The drawing under review shows one solid part. Ordinate dimensions are in mm from its lowest x, y, z. A direction names the side the tool comes from. Round coordinates to 2 decimals unless told otherwise and drop trailing zeros. Order: outer loops, then holes, each group sorted by start corner. A loop starts at its lowest first (then second) coordinate and runs counter-clockwise, first axis right, second up. Notation, with made-up numbers: (7.25, -24.5) -> (54.25, -24.5) arc R26 cw to (54.25, -6.5) -> close; hole circle Ø10 at (71, 0.25). An arc over 180 degrees is marked (long way). Put each result on its own line as item: value. Start each with the question number.
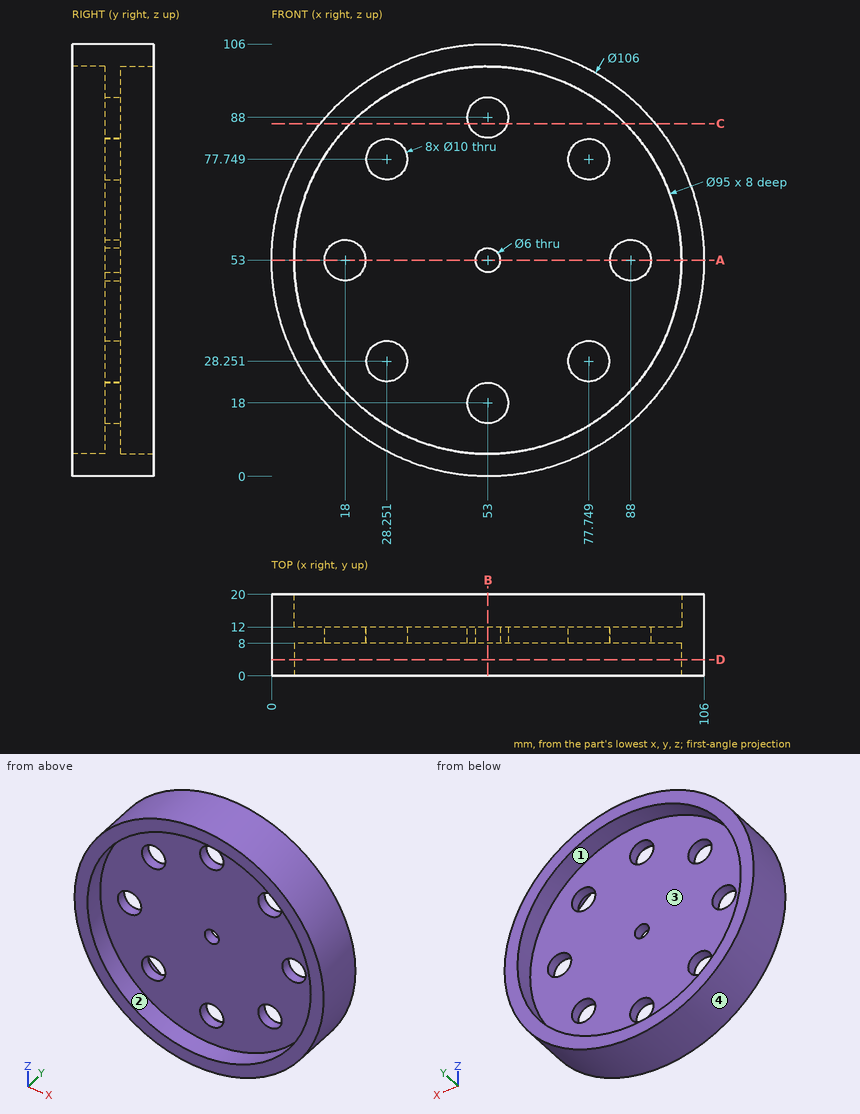
Item 1: Tool access review of the marked faces 1 and 2: name each direction out of +Z, -Z, +X, -X, +Y, -Y from which nothing blocks a thin tool from reaching the whole face with its end or side.
Item 2: Consider section B-B, the plane x = 53. Write out the cut boundary in (y, z).
Item 3: Consider section D-D, the plane y = 4. Write out the cut boundary in (x, z), plus the area to 3 significant figures.
Item 4: Mouldability with a two-part tool opening along X and no side actions: class the marked faces 3 and 4 as +X half, -X half, draft (parallel to the pull), parting line (faces both ways), or undercut.
Item 5: Consider section C-C, the plane z = 86.5. Write out the cut boundary in (x, y) (1 decimal).
Item 6: Consider section A-A, the plane z = 53. Write out the cut boundary in (x, y), plus the area to 3 significant figures.
Item 7: For L1, parallel to Z at x = 53, y = 9.15; L2, parallel to Z at x = 54, y = 17.5, list the stretches that pass through material, from the lowest coordinate up.
Item 8: Insertion check: pin 1 Ø6 at (y, z) = (13.5, 93) entering from -X; pin 2 Ø5 at (y, z) = (14, 24.5) entering from -X (1 decimal); pin 3 Ø7 at (x, z) = (53, 53) entering from +Y. Each pin has a flat end and moves straight along its axis. Give the tip position at first contact, or say it passes through.
Evaluation:
1. face 1: +Y
1. face 2: -Y
2. outline: (0, 0) -> (20, 0) -> (20, 5.5) -> (12, 5.5) -> (12, 13) -> (8, 13) -> (8, 5.5) -> (0, 5.5) -> close; (0, 100.5) -> (8, 100.5) -> (8, 93) -> (12, 93) -> (12, 100.5) -> (20, 100.5) -> (20, 106) -> (0, 106) -> close; (8, 23) -> (12, 23) -> (12, 50) -> (8, 50) -> close; (8, 56) -> (12, 56) -> (12, 83) -> (8, 83) -> close
3. outline: circle Ø106 at (53, 53); hole circle Ø95 at (53, 53)
3. area: 1,740 mm^2
4. face 3: undercut
4. face 4: parting line
5. outline: (11.9, 0) -> (19.3, 0) -> (19.3, 8) -> (48.2, 8) -> (48.2, 12) -> (19.3, 12) -> (19.3, 20) -> (11.9, 20) -> close; (57.8, 8) -> (86.7, 8) -> (86.7, 0) -> (94.1, 0) -> (94.1, 20) -> (86.7, 20) -> (86.7, 12) -> (57.8, 12) -> close
6. outline: (0, 0) -> (5.5, 0) -> (5.5, 8) -> (13, 8) -> (13, 12) -> (5.5, 12) -> (5.5, 20) -> (0, 20) -> close; (23, 8) -> (50, 8) -> (50, 12) -> (23, 12) -> close; (56, 8) -> (83, 8) -> (83, 12) -> (56, 12) -> close; (93, 8) -> (100.5, 8) -> (100.5, 0) -> (106, 0) -> (106, 20) -> (100.5, 20) -> (100.5, 12) -> (93, 12) -> close
6. area: 496 mm^2
7. L1: z = 0 to 13, 23 to 50, 56 to 83, 93 to 106
7. L2: z = 0.01 to 5.51, 100.49 to 105.99
8. pin 1: stops at x = 15.05
8. pin 2: stops at x = 6.8
8. pin 3: stops at y = 12
